The figure shows three views and two pictorial views of one solid part (mm, origin at its lowest corner). Answer the questions. A direction names the side the tool comes from. Round coordinates to 2 decimals unless told otherwise and drop trailing zeros. Order: outer loops, then holes, each group sorted by start corner. A loop starts at its lowest first (then second) coordinate and runs counter-clockwise, first axis right, second up. Notation, with made-up numbers: (38, 66) - (74, 66) arc R21 ccw to (74, 102) - close; hole circle Ø8 at (83.5, 38). An arc over 180 degrees is marked (long way). Answer as a JSON object with one key per item and string values. Group by question number.
Q1. A tool of negligible diameter and unlimited length cuts with its end or side. For the marked faces 4, 5 and 6, from which of +Z, -Z, +X, -X, +Y, -Y can it reach the whole face along a straight path? Write none if from no direction.
Q2. A cutting plane is placed at A-A on x = 30. Determine the outline of the cut face in (y, z), and give its area (3 significant figures).
Q3. A cutting plane is placed at C-C on z = 23.5. Determine the outline of the cut face in (x, y).
Q4. Given pin 1 Ø2 at (y, z) = (8.5, 7.5) entering from +X; pin 2 Ø1 at (x, y) = (1, 9.5) entering from -Z; pin 3 Ø2.5 at (x, z) = (35, 46) entering from -Y, each flat-ended and moving along its own axis, determine where each tip first touches the part or whether it passes through.
Q5. The mould has two halves that part along X. Classify the marked faces 1, 2 and 3: pulls with the +X half, pulls with the -X half, needs draft (parallel to the pull), parting line crosses it, or undercut.
Q6. Consider line 1 (Z direction, x = 35, y = 11); line 2 (Y direction, x = 21, z = 14); line 3 (Y direction, x = 5.5, z = 22.5). Determine where each line is inside the solid, lowest interval first.
Q7. A cutting plane is placed at B-B on y = 10. Determine the outline of the cut face in (x, z).
Q8. A cutting plane is placed at D-D on y = 16.5. Determine the outline of the cut face in (x, z), and give its area (3 significant figures).
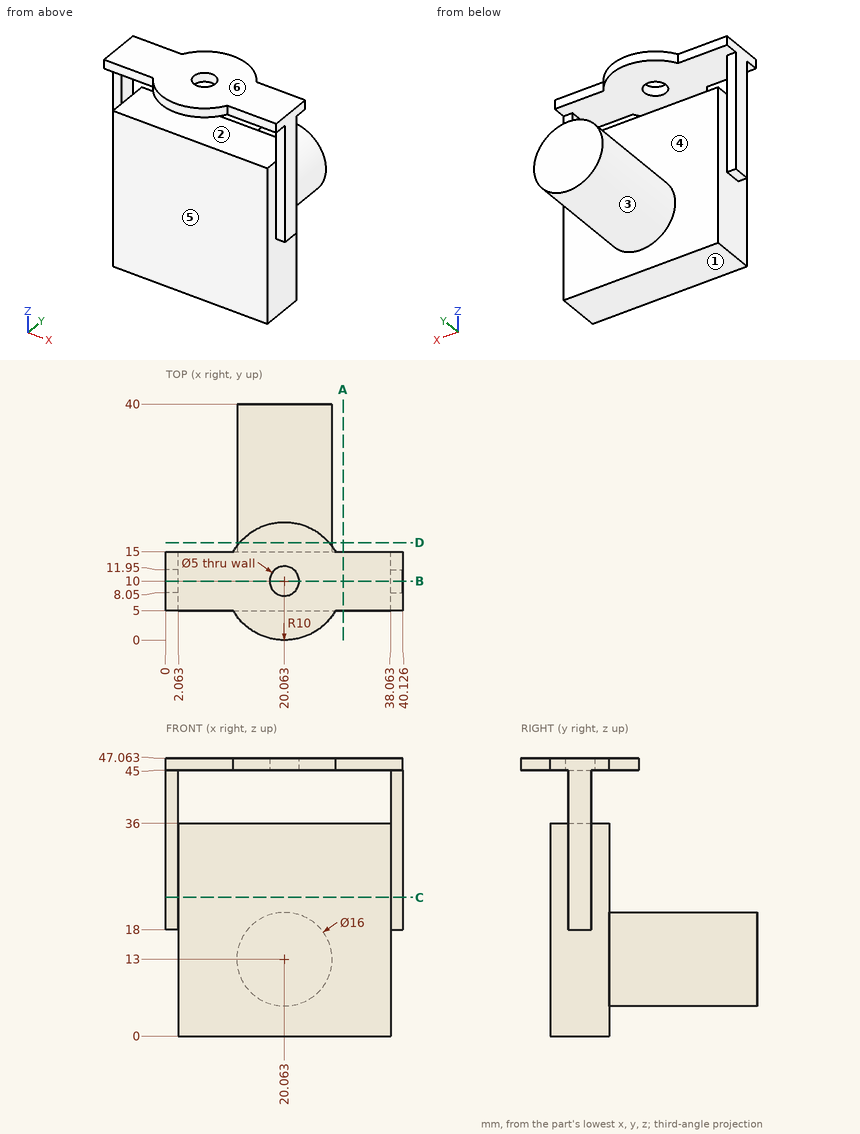
Result set:
{
 "1": {"face 4": "+Y", "face 5": "-Z, +X, -X, -Y", "face 6": "+Z, +X, -X, +Y, -Y"},
 "2": {"outline": "(5, 0) - (15, 0) - (15, 36) - (5, 36) - close; (5, 45) - (15, 45) - (15, 47.06) - (5, 47.06) - close", "area": "381 mm²"},
 "3": {"outline": "(0, 8.05) - (2.06, 8.05) - (2.06, 5) - (38.06, 5) - (38.06, 8.05) - (40.13, 8.05) - (40.13, 11.95) - (38.06, 11.95) - (38.06, 15) - (2.06, 15) - (2.06, 11.95) - (0, 11.95) - close"},
 "4": {"pin 1": "stops at x = 38.06", "pin 2": "stops at z = 18", "pin 3": "stops at y = 5"},
 "5": {"face 1": "needs draft", "face 2": "undercut", "face 3": "parting line crosses it"},
 "6": {"line 1": "z = 0 to 36, 45 to 47.06", "line 2": "y = 5 to 40", "line 3": "y = 5 to 15"},
 "7": {"outline": "(0, 18) - (2.06, 18) - (2.06, 0) - (38.06, 0) - (38.06, 18) - (40.13, 18) - (40.13, 47.06) - (22.56, 47.06) - (22.56, 45) - (38.06, 45) - (38.06, 36) - (2.06, 36) - (2.06, 45) - (17.56, 45) - (17.56, 47.06) - (0, 47.06) - close"},
 "8": {"outline": "circle Ø16 at (20.06, 13); (12.46, 45) - (27.66, 45) - (27.66, 47.06) - (12.46, 47.06) - close", "area": "232 mm²"}
}
